```python
from build123d import *

# Parameters (mm, degrees)
F0_W     = 141
F0_H     = 140
F1_DEPTH = 135
F3_R     = 9
F2_W     = 20
F2_H     = 10
F4_DEPTH = 50
F2_W_2   = 15
F2_H_2   = 2
F5_DEPTH = 25


with BuildPart() as f1:
    # F0 (on Top) → F1 (new body)
    with BuildSketch(Plane.XY):
        with Locations((70.5, 70)):
            Rectangle(F0_W, F0_H)
    extrude(amount=F1_DEPTH)

    # F3
    f3_edges = [f1.edges().sort_by_distance(p)[0] for p in [
        (70.5, 140, 0),
        (70.5, 140, 135),
        (70.5, 0, 0),
        (70.5, 0, 135),
    ]]
    fillet(f3_edges, radius=F3_R)

    # F2 (on face) → F4 (join)
    with BuildSketch(Plane.YZ.offset(141)):
        with Locations((123, 12)):
            Rectangle(F2_W, F2_H)
    extrude(amount=F4_DEPTH)

    # F2 (on face) → F5 (join)
    with BuildSketch(Plane.YZ.offset(141)):
        with Locations((95.5, 8)):
            Rectangle(F2_W_2, F2_H_2)
    extrude(amount=F5_DEPTH)


solid = f1.part
```
Design review of the part built by this model. Coordinates are the model's own, in mm. A direction names the side the tool comes from. Coordinates: 2 decimals unless noted, no trailing zeros. Write each loop counter-clockwise with the first axis right and the second up, starting at its lowest first coordinate (ties: lowest second). Pieces come first, ordered by that corner, then holes. Notation, with made-up numbers: M 15.25,84.5 L 51.25,84.5 A22 cw 51.25,106.5 Z; hole C 68.25,32 d4. An arc over 180 degrees is marked long. Answer as a JSON object with one key per item and string values.
Item 1: Machinability: for faces 1 (the flat face through (166, 133, 12)), 2 (the flat face through (153, 95, 7)), 3 (the flat face through (153, 95, 9)), 4 (the flat face through (166, 113, 12)), which of the approach directions +Z, -Z, +X, -X, +Y, -Y give a long, thin tool a straight path to every point of the face, cutting with its end or side? Answer none if there is none.
Outcome:
{"face 1": "+Z, -Z, +X, +Y", "face 2": "-Z, +X, +Y, -Y", "face 3": "+Z, +X, -Y", "face 4": "+Z, -Z, +X"}
Item 2: Add section A-A, the plane x = 144. Give the boundary of the cut face in (y, z).
Outcome:
{"outline": "M 88,7 L 103,7 L 103,9 L 88,9 Z; M 113,7 L 133,7 L 133,17 L 113,17 Z"}
Item 3: Add section C-C, the plane y = 42. Give the boundary of the cut face in (x, z), and give its area (3 significant figures).
Outcome:
{"outline": "M 0,0 L 141,0 L 141,135 L 0,135 Z", "area": "19,000 mm²"}
Item 4: Insertion check: pin 1 Ø22 at (x, y) = (156.5, 122.5) entering from -Z; pin 2 Ø1 at (y, z) = (58.5, 94) entering from +X; pin 3 Ø8 at (x, z) = (163, 12.5) entering from +Y. Each pin has a flat end and moves straight along its axis. Give the tip position at first contact, or say it passes through.
Outcome:
{"pin 1": "z = 7", "pin 2": "x = 141", "pin 3": "y = 133"}
Item 5: Add section B-B, the plane z = 46. Give the boundary of the cut face in (x, y), and give its area (3 significant figures).
Outcome:
{"outline": "M 0,0 L 141,0 L 141,140 L 0,140 Z", "area": "19,700 mm²"}
Item 6: Wall thickness on probe 1 along X at (y, z) = (23, 37); probe 2 along Z at (x, y) = (105.5, 133); probe 3 along Y at (x, z) = (12, 5): over which ranges is each line inside the solid? List them lowest first.
Outcome:
{"probe 1": "0 to 141", "probe 2": "0.23 to 134.77", "probe 3": "0.94 to 139.06"}
